```python
from build123d import *

# Parameters (mm, degrees)
F0_W     = 50.8
F0_H     = 50.8
F0_R     = 14.889402
F1_DEPTH = 50.8
F2_W     = 25.4
F2_H     = 25.4
F3_DEPTH = 12.7
F4_R     = 12.7
F5_DEPTH = 12.7


with BuildPart() as f1:
    # F0 (on Front) → F1 (new body)
    with BuildSketch(Plane.XZ):
        with Locations((-25.4, -25.4)):
            Rectangle(F0_W, F0_H)
        with Locations((-25.4, -25.4)):
            Circle(F0_R, mode=Mode.SUBTRACT)
    extrude(amount=F1_DEPTH)

    # F2 (on face) → F3 (join)
    with BuildSketch(Plane(origin=(-50.8, 0, 0), x_dir=(0, -1, 0), z_dir=(-1, 0, 0))):
        with Locations((25.4, -25.4)):
            Rectangle(F2_W, F2_H)
    extrude(amount=F3_DEPTH)

    # F4 (on face) → F5 (join)
    with BuildSketch(Plane.XY):
        with Locations((-25.4, -25.4)):
            Circle(F4_R)
    extrude(amount=F5_DEPTH)


solid = f1.part
```
For this review, take the finished solid that the model builds, in its own axes (mm). A direction names the side the tool comes from. Round coordinates to 2 decimals unless told otherwise and drop trailing zeros. Order: outer loops, then holes, each group sorted by start corner. A loop starts at its lowest first (then second) coordinate and runs counter-clockwise, first axis right, second up.
Q1. We need section C-C, the plane x = -25.4. Give the boundary of the cut face in (y, z).
Findings below:
outline: (-50.8, -50.8) - (0, -50.8) - (0, -40.29) - (-50.8, -40.29) - close; (-50.8, -10.51) - (0, -10.51) - (0, 0) - (-12.7, 0) - (-12.7, 12.7) - (-38.1, 12.7) - (-38.1, 0) - (-50.8, 0) - close
Q2. We need section A-A, the plane z = -25.4. Give the boundary of the cut face in (x, y).
Findings below:
outline: (-63.5, -38.1) - (-50.8, -38.1) - (-50.8, -50.8) - (-40.29, -50.8) - (-40.29, 0) - (-50.8, 0) - (-50.8, -12.7) - (-63.5, -12.7) - close; (-10.51, -50.8) - (0, -50.8) - (0, 0) - (-10.51, 0) - close
Q3. Machinability: for faces 5 (the flat face through (-57, -38.1, -26)), 6 (the flat face through (-57, -25, -12.7)), 7 (the cylindrical face through (-28.15, -37.8, 6.26)), which of the approach directions +Z, -Z, +X, -X, +Y, -Y give a long, thin tool a straight path to every point of the face, cutting with its end or side? Answer none if there is none.
Findings below:
face 5: +Z, -Z, -X, -Y
face 6: +Z, -X, +Y, -Y
face 7: +Z
Q4. We need section D-D, the plane y = -36. Give the boundary of the cut face in (x, z) (3 decimals), plus the area to 3 significant figures.
Findings below:
outline: (-63.5, -38.1) - (-50.8, -38.1) - (-50.8, -50.8) - (0, -50.8) - (0, 0) - (-18.405, 0) - (-18.405, 12.7) - (-32.395, 12.7) - (-32.395, 0) - (-50.8, 0) - (-50.8, -12.7) - (-63.5, -12.7) - close; hole circle Ø29.779 at (-25.4, -25.4)
area: 2,380 mm2
Q5. Insertion check: P1, Ø6.5, axis at x = -56.5, y = -21, coming from the -Z side; P2, Ø8, axis at y = -16, z = -3, coming from the -X side; P3, Ø6.5, axis at x = -57, z = -27.5, coming from the -Y side; P4, Ø18, axis at x = -25.4, z = -25.4, coming from the +Y side. Each pin has a flat end and moves straight along its axis. Give the tip position at first contact, or say it passes through.
Findings below:
P1: stops at z = -38.1
P2: stops at x = -50.8
P3: stops at y = -38.1
P4: passes through
Q6. We need section B-B, the plane y = -25.4. Give the boundary of the cut face in (x, z).
Findings below:
outline: (-63.5, -38.1) - (-50.8, -38.1) - (-50.8, -50.8) - (0, -50.8) - (0, 0) - (-12.7, 0) - (-12.7, 12.7) - (-38.1, 12.7) - (-38.1, 0) - (-50.8, 0) - (-50.8, -12.7) - (-63.5, -12.7) - close; hole circle Ø29.78 at (-25.4, -25.4)
Q7. Wall thickness on line 1 (X direction, y = -23, z = -25); line 2 (Z direction, x = -25, y = -24); line 3 (X direction, y = -11, z = -25): over which ranges is each line inside the solid? List them lowest first.
Findings below:
line 1: x = -63.5 to -40.28, -10.52 to 0
line 2: z = -50.8 to -40.28, -10.52 to 12.7
line 3: x = -50.8 to -40.28, -10.52 to 0
Q8. Mouldability with a two-part tool opening along Z and no side actions: class faces 1 (the flat face through (-31.4, -13.8, 0)), 2 (the flat face through (-57, -25, -38.1)), 3 (the flat face through (-57, -12.7, -26)), 4 (the cylindrical face through (-18.53, -25.04, -38.61)) as pulls with the +Z half, pulls with the -Z half, needs draft (parallel to the pull), parting line crosses it, or undercut.
Findings below:
face 1: pulls with the +Z half
face 2: pulls with the -Z half
face 3: needs draft
face 4: undercut
